Design review of the part built by this model. Coordinates are the model's own, in mm. A direction names the side the tool comes from. Give positions to 0.01 mm unless a question says otherwise; leave off trailing zeros. Write each loop counter-clockwise with the first axis right and the second up, starting at its lowest first coordinate (ties: lowest second). Pieces come first, ordered by that corner, then holes.
```python
from build123d import *

# Parameters (mm, degrees)
BOSS_EXTRUDE1_DEPTH = 24
SKETCH4_R           = 1.55
CUT_EXTRUDE1_DEPTH  = 8


with BuildPart() as part:
    # Sketch3 → Boss-Extrude1 (new, symmetric)
    with BuildSketch(Plane.XY):
        Polygon((0, 5.773502692), (5, 2.886751346), (5, -2.886751346), (0, -5.773502692), (-5, -2.886751346), (-5, 2.886751346), align=None)
    extrude(amount=BOSS_EXTRUDE1_DEPTH, both=True)

    # Sketch4 → Cut-Extrude1 (cut)
    with BuildSketch(Plane.XY.offset(24)):
        with BuildLine():
            Line((-5, -2.886751346), (-2.500000044, -4.330126993))
            ThreePointArc((-2.500000044, -4.330126993), (-3.298726627, -3.757446293), (-3.97, -3.039588788))
            Line((-3.97, -3.039588788), (-3.97, 3.039588788))
            ThreePointArc((-3.97, 3.039588788), (-3.298726623, 3.757446296), (-2.500000037, 4.330126998))
            Line((-2.500000037, 4.330126998), (-5, 2.886751346))
            Line((-5, 2.886751346), (-5, -2.886751346))
        make_face()
        with BuildLine():
            ThreePointArc((-2.500000037, 4.330126998), (-7.5e-08, 5), (2.499999906, 4.330127073))
            Line((2.499999906, 4.330127073), (0, 5.773502692))
            Line((0, 5.773502692), (-2.500000037, 4.330126998))
        make_face()
        with BuildLine():
            Line((3.97, 3.039588788), (3.97, -3.039588788))
            ThreePointArc((3.97, -3.039588788), (3.298726555, -3.757446356), (2.499999878, -4.330127089))
            Line((2.499999878, -4.330127089), (5, -2.886751346))
            Line((5, -2.886751346), (5, 2.886751346))
            Line((5, 2.886751346), (2.499999906, 4.330127073))
            ThreePointArc((2.499999906, 4.330127073), (3.298726567, 3.757446345), (3.97, 3.039588788))
        make_face()
        with BuildLine():
            Line((0, -5.773502692), (2.499999878, -4.330127089))
            ThreePointArc((2.499999878, -4.330127089), (-9.6e-08, -5), (-2.500000044, -4.330126993))
            Line((-2.500000044, -4.330126993), (0, -5.773502692))
        make_face()
        Circle(SKETCH4_R)
    extrude(amount=-CUT_EXTRUDE1_DEPTH, mode=Mode.SUBTRACT)


solid = part.part
```
(1) Consider section A-A, the plane y = 0. Give the boundary of the cut face in (x, z), then the cut area to 3 significant figures.
Resolved:
outline: (-5, -24) - (5, -24) - (5, 16) - (3.97, 16) - (3.97, 24) - (1.55, 24) - (1.55, 16) - (-1.55, 16) - (-1.55, 24) - (-3.97, 24) - (-3.97, 16) - (-5, 16) - close
area: 439 mm2
(2) To check wall thickness, follow L1, parallel to Y at x = 0, z = 18.25; L2, parallel to Z at x = -0.5, y = -1.25; L3, parallel to X at y = -1.25, z = 22. State the ranges of each line that lie inside material, in increasing order.
Resolved:
L1: y = -5 to -1.55, 1.55 to 5
L2: z = -24 to 16
L3: x = -3.97 to -0.92, 0.92 to 3.97
(3) Mouldability with a two-part tool opening along X and no side actions: class faces 1 (the face through (0.715, -1.375, 20.056)), 2 (the face through (-5, 0, -4)), 3 (the face through (0, 0, 16)), 4 (the face through (3.97, 0, 20)) as pulls with the +X half, pulls with the -X half, needs draft (parallel to the pull), parting line crosses it, or undercut.
Resolved:
face 1: undercut
face 2: pulls with the -X half
face 3: undercut
face 4: pulls with the +X half
(4) Consider section C-C, the plane x = 0.5. Give the boundary of the cut face in (y, z).
Resolved:
outline: (-5.48, -24) - (5.48, -24) - (5.48, 16) - (4.97, 16) - (4.97, 24) - (1.47, 24) - (1.47, 16) - (-1.47, 16) - (-1.47, 24) - (-4.97, 24) - (-4.97, 16) - (-5.48, 16) - close
(5) Clearance check with flat-ended pins moving along their axes: P1, Ø1, axis at x = 1.5, z = 9.5, coming from the +Y side; P2, Ø0.8, axis at x = 4.5, y = -1.5, coming from the +Z side; P3, Ø6, axis at x = -2, z = 4.5, coming from the +Y side. State where each tip first meets the part, or that it passes through.
Resolved:
P1: stops at y = 5.2
P2: stops at z = 16
P3: stops at y = 5.77
(6) Consider section B-B, the plane z = -8. Give the boundary of the cut face in (x, y).
Resolved:
outline: (-5, -2.89) - (0, -5.77) - (5, -2.89) - (5, 2.89) - (0, 5.77) - (-5, 2.89) - close
(7) Tool access review of faces 5 (the face through (0, -5.2, 16)), 6 (the face through (-2.535, 4.31, -3.72)), 7 (the face through (-3.97, 0, 20)): name each direction out of +Z, -Z, +X, -X, +Y, -Y from which nothing blocks a thin tool from reaching the whole face with its end or side.
Resolved:
face 5: +Z, -Y
face 6: +Z, -Z, -X, +Y
face 7: +Z, -X, +Y, -Y
